Autodesk Inventor part; units mm, degrees
ref_plane "YZ Plane" through (0, 0, 0) normal (1, 0, 0) x (0, 1, 0)
ref_plane "XZ Plane" through (0, 0, 0) normal (0, 1, 0) x (-1, 0, 0)
ref_plane "XY Plane" through (0, 0, 0) normal (0, 0, 1) x (1, 0, 0)
sketch "Sketch1" plane through (0, 0, 0) normal (0, 0, 1) x (1, 0, 0)
  circle A0 centre (0, 0) radius 30
  dimension "d0" = 60
extrude "Extrusion1" add sketch "Sketch1" along normal blind 30
sketch "Sketch2" plane through (0, 0, 30) normal (0, 0, 1) x (1, 0, 0)
  circle A0 centre (0, 0) radius 26
  dimension "d3" = 52
extrude "Extrusion2" cut sketch "Sketch2" against normal blind 10
sketch "Sketch3" plane through (0, 0, 0) normal (0, 0, -1) x (-1, 0, 0)
  circle A0 centre (0, 0) radius 26
  dimension "d6" = 52
extrude "Extrusion3" cut sketch "Sketch3" against normal blind 10
sketch "Sketch4" plane through (0, 0, 10) normal (0, 0, -1) x (-1, 0, 0)
  circle A0 centre (0, 0) radius 15
  dimension "d9" = 30
extrude "Extrusion4" add sketch "Sketch4" along normal blind 10
sketch "Sketch5" plane through (0, 0, 20) normal (0, 0, 1) x (1, 0, 0)
  circle A0 centre (0, 0) radius 15
  dimension "d12" = 30
extrude "Extrusion5" add sketch "Sketch5" along normal blind 10
sketch "Sketch6" plane through (0, 0, 30) normal (0, 0, 1) x (1, 0, 0)
  circle A0 centre (0, 0) radius 10
  dimension "d15" = 20
extrude "Extrusion6" cut sketch "Sketch6" against normal blind 30
properties part number "4 - Part 3"
The model under review builds one solid part; all positions refer to its coordinate system, in mm. A direction names the side the tool comes from. Give positions to 0.01 mm unless a question says otherwise; leave off trailing zeros. Write each loop counter-clockwise with the first axis right and the second up, starting at its lowest first coordinate (ties: lowest second). Pieces come first, ordered by that corner, then holes.
1. Add section A-A, the plane x = 0. Write out the cut boundary in (y, z).
2. For P1, Ø5, axis at x = 16, z = 16.5, coming from the +Y side; P2, Ø5, axis at x = 15, z = 9, coming from the -Y side; P3, Ø1.5, axis at x = 22.5, y = 23.5, coming from the +Z side; P4, Ø6, axis at x = 2, z = 4.5, coming from the +Y side, all flat-tipped, find the tip position at first contact; note any pin that passes through.
3. Tool access review of faces 1 (the cylindrical face through (-14.985, -0.66, 24.93)), 2 (the cylindrical face through (-2.17, -9.76, 15.21)), 3 (the cylindrical face through (14.985, -0.66, 5.07)): name each direction out of +Z, -Z, +X, -X, +Y, -Y from which nothing blocks a thin tool from reaching the whole face with its end or side.
4. Add section D-D, the plane z = 15.5. Write out the cut boundary in (x, y), plus the area to 3 significant figures.
5. Wall thickness on L1, parallel to Y at x = 0, z = 26.25; L2, parallel to X at y = 11.5, z = 27.5; L3, parallel to Y at x = 6.5, z = 25.75: over which ranges is each line inside the solid? List them lowest first.
6. Add section C-C, the plane z = 28.25. Write out the cut boundary in (x, y), plus the area to 3 significant figures.
7. Draft analysis for pull direction X (two halves, no side actions). For faces 4 (the cylindrical face through (-29.97, -1.32, 14.79)), 5 (the flat face through (3, -10, 30)), 6 (the flat face through (11, -11, 20)), state which applies: +X half, -X half, draft (parallel to the pull), parting line (faces both ways), or undercut.
Worked answers:
1. outline: (-30, 0) - (-26, 0) - (-26, 10) - (-15, 10) - (-15, 0) - (-10, 0) - (-10, 30) - (-15, 30) - (-15, 20) - (-26, 20) - (-26, 30) - (-30, 30) - close; (10, 0) - (15, 0) - (15, 10) - (26, 10) - (26, 0) - (30, 0) - (30, 30) - (26, 30) - (26, 20) - (15, 20) - (15, 30) - (10, 30) - close
2. P1: stops at y = 26.79
2. P2: stops at y = -27.27
2. P3: passes through
2. P4: stops at y = 30
3. face 1: +Z
3. face 2: +Z, -Z
3. face 3: -Z
4. outline: circle Ø60 at (0, 0); hole circle Ø20 at (0, 0)
4. area: 2,510 mm2
5. L1: y = -30 to -26, -15 to -10, 10 to 15, 26 to 30
5. L2: x = -27.71 to -23.32, -9.63 to 9.63, 23.32 to 27.71
5. L3: y = -29.29 to -25.17, -13.52 to -7.6, 7.6 to 13.52, 25.17 to 29.29
6. outline: circle Ø60 at (0, 0); circle Ø30 at (0, 0); hole circle Ø52 at (0, 0); hole circle Ø20 at (0, 0)
6. area: 1,100 mm2
7. face 4: parting line
7. face 5: draft
7. face 6: undercut
